Here's how the part is built. I have some questions about the finished solid (model axes, mm). Face numbers are marked on the shaded views. A direction names the side the tool comes from. Coordinates: 2 decimals unless noted, no trailing zeros. Loops run counter-clockwise (first coordinate to the right, second up) from the corner with the lowest first, then second, coordinate; pieces in that order, holes last. Notation, with made-up numbers: M -35.5,-21.75 L -17.5,-21.75 A28 ccw -17.5,-2.75 Z; hole C 64.25,54.5 d5. An arc over 180 degrees is marked long. Use CSV: the item, a comma, the result in double quotes. Start each with the question number.
Q1. If we section it at D-D (z = 9.5): State how many separate pieces and enclosed holes the cut face has, and give its area (3 significant figures).
Q2. Which directions (+Z, -Z, +X, -X, +Y, -Y) give clear straight access to the entire face, cutting with the end or side of a thin tool? Please do the marked faces 1 and 2.
Q3. For pin 1 Ø12 at (x, y) = (-23, -35.5) entering from -Z; pin 2 Ø0.6 at (x, z) = (-45.5, 20) entering from -Y (3 decimals); pin 3 Ø0.8 at (y, z) = (-37.5, 11) entering from -X (3 decimals), each with a flat end and sliding along its axis, tell me the tip position at first contact or that it passes through.
Q4. If we section it at B-B (y = -53.65): Please give me the cut outline in (x, z) (3 decimals).
Q5. If we section it at C-C (x = -17): Please give me the cut outline in (y, z), and give its area (3 significant figures).
Q6. If we section it at A-A (x = 32): Please give me the cut outline in (y, z), and give its area (3 significant figures).
Q7. Please list where these lines run through material, in increasing order: probe 1 along X at (y, z) = (-30, 16.5) (3 decimals); probe 2 along X at (y, z) = (-53, 20) (3 decimals); probe 3 along Y at (x, z) = (19, 4). Write a range as [from, to].
Q8. If we mould it in two halves opening along X, with no side actions, what happens to the marked faces 3, 4 and 5? For each: +X half, -X half, draft (parallel to the pull), parting line (faces both ways), or undercut.
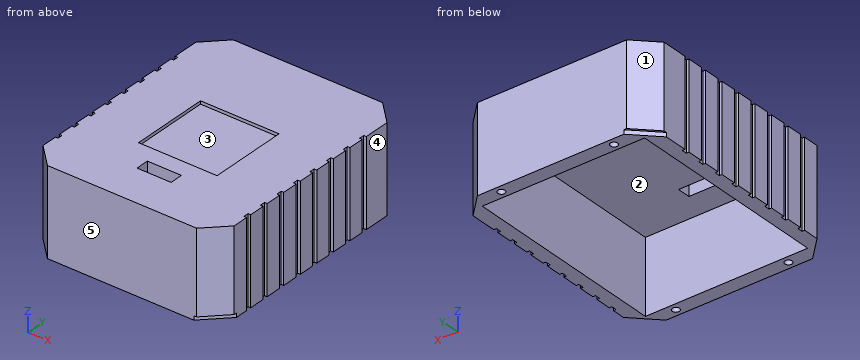
from build123d import *

# Parameters (mm, degrees)
SKETCH1_W           = 92.71
SKETCH1_H           = 114.3
BOSS_EXTRUDE1_DEPTH = 41.91
SKETCH2_W           = 2.54
SKETCH2_H           = 2.54
CUT_EXTRUDE1_DEPTH  = 85.683862837
CHAMFER1_SIZE       = 10.16
SKETCH3_R           = 1.750000056
CUT_EXTRUDE2_DEPTH  = 25.4
SKETCH4_W           = 78.71
SKETCH4_H           = 100.30000006
CUT_EXTRUDE3_DEPTH  = 35.56
SKETCH6_W           = 16.51
SKETCH6_H           = 6.35
CUT_EXTRUDE5_DEPTH  = 85.683862837
CUT_EXTRUDE6_DEPTH  = 2
SKETCH8_W           = 38.1
SKETCH8_H           = 38.1
CUT_EXTRUDE7_DEPTH  = 1.5


with BuildPart() as part:
    # Sketch1 → Boss-Extrude1 (new body)
    with BuildSketch(Plane.XY):
        Rectangle(SKETCH1_W, SKETCH1_H)
    extrude(amount=BOSS_EXTRUDE1_DEPTH)

    # Sketch2 → Cut-Extrude1 (cut, through all)
    with BuildSketch(Plane(origin=(0, 0, 0), x_dir=(-1, 0, 0), z_dir=(0, 0, -1))):
        with Locations((-46.355, -38.1)):
            Rectangle(SKETCH2_W, SKETCH2_H)
        with Locations((46.355, -38.1)):
            Rectangle(SKETCH2_W, SKETCH2_H)
        with Locations((-46.355, -27.94)):
            Rectangle(SKETCH2_W, SKETCH2_H)
        with Locations((46.355, -27.94)):
            Rectangle(SKETCH2_W, SKETCH2_H)
        with Locations((-46.355, -17.78)):
            Rectangle(SKETCH2_W, SKETCH2_H)
        with Locations((46.355, -17.78)):
            Rectangle(SKETCH2_W, SKETCH2_H)
        with Locations((-46.355, -7.62)):
            Rectangle(SKETCH2_W, SKETCH2_H)
        with Locations((46.355, -7.62)):
            Rectangle(SKETCH2_W, SKETCH2_H)
        with Locations((-46.355, 2.54)):
            Rectangle(SKETCH2_W, SKETCH2_H)
        with Locations((46.355, 2.54)):
            Rectangle(SKETCH2_W, SKETCH2_H)
        with Locations((-46.355, 12.7)):
            Rectangle(SKETCH2_W, SKETCH2_H)
        with Locations((46.355, 12.7)):
            Rectangle(SKETCH2_W, SKETCH2_H)
        with Locations((-46.355, 22.86)):
            Rectangle(SKETCH2_W, SKETCH2_H)
        with Locations((46.355, 22.86)):
            Rectangle(SKETCH2_W, SKETCH2_H)
        with Locations((-46.355, 33.02)):
            Rectangle(SKETCH2_W, SKETCH2_H)
        with Locations((46.355, 33.02)):
            Rectangle(SKETCH2_W, SKETCH2_H)
    extrude(amount=-CUT_EXTRUDE1_DEPTH, mode=Mode.SUBTRACT)

    # Chamfer1
    chamfer1_edges = [part.edges().sort_by_distance(p)[0] for p in [
        (46.355, -57.15, 20.955),
        (-46.355, -57.15, 20.955),
        (-46.355, 57.15, 20.955),
        (46.355, 57.15, 20.955),
    ]]
    chamfer(chamfer1_edges, length=CHAMFER1_SIZE)

    # Sketch3 → Cut-Extrude2 (cut)
    with BuildSketch(Plane(origin=(0, 0, 0), x_dir=(-1, 0, 0), z_dir=(0, 0, -1))):
        with Locations((-27.305, -53.649999888)):
            Circle(SKETCH3_R)
        with Locations((-27.305, 53.65)):
            Circle(SKETCH3_R)
        with Locations((27.305, 53.649999888)):
            Circle(SKETCH3_R)
        with Locations((27.305, -53.649999888)):
            Circle(SKETCH3_R)
    extrude(amount=-CUT_EXTRUDE2_DEPTH, mode=Mode.SUBTRACT)

    # Sketch4 → Cut-Extrude3 (cut)
    with BuildSketch(Plane(origin=(0, 0, 0), x_dir=(-1, 0, 0), z_dir=(0, 0, -1))):
        Rectangle(SKETCH4_W, SKETCH4_H)
    extrude(amount=-CUT_EXTRUDE3_DEPTH, mode=Mode.SUBTRACT)

    # Sketch6 → Cut-Extrude5 (cut, through all)
    with BuildSketch(Plane.XY.offset(41.91)):
        with Locations((0, -34.29)):
            Rectangle(SKETCH6_W, SKETCH6_H)
    extrude(amount=-CUT_EXTRUDE5_DEPTH, mode=Mode.SUBTRACT)

    # Sketch7 → Cut-Extrude6 (cut)
    with BuildSketch(Plane(origin=(0, 0, 0), x_dir=(-1, 0, 0), z_dir=(0, 0, -1))):
        Polygon((40.567893219, 51.362893219), (46.355, 45.575786438), (46.355, 46.99), (36.195, 57.15), (34.780786438, 57.15), align=None)
        Polygon((-40.567893219, -51.362893219), (-46.355, -45.575786438), (-46.355, -46.99), (-36.195, -57.15), (-34.780786438, -57.15), align=None)
    extrude(amount=-CUT_EXTRUDE6_DEPTH, mode=Mode.SUBTRACT)

    # Sketch8 → Cut-Extrude7 (cut)
    with BuildSketch(Plane.XY.offset(41.91)):
        with Locations((0, -3.81)):
            Rectangle(SKETCH8_W, SKETCH8_H)
    extrude(amount=-CUT_EXTRUDE7_DEPTH, mode=Mode.SUBTRACT)


solid = part.part
Results below:
1,separate pieces,"1"
1,enclosed holes,"5"
1,area,"2,410 mm^2"
2,face 1,"+Z, -Z, -X, +Y"
2,face 2,"-Z"
3,pin 1,"z = 35.56"
3,pin 2,"y = -48.145"
3,pin 3,"x = -45.085"
4,outline,"M -39.695,0 L -29.055,0 L -29.055,25.4 L -25.555,25.4 L -25.555,0 L 25.555,0 L 25.555,25.4 L 29.055,25.4 L 29.055,0 L 38.281,0 L 38.281,2 L 39.695,2 L 39.695,41.91 L -39.695,41.91 Z"
5,outline,"M -57.15,0 L -50.15,0 L -50.15,35.56 L 50.15,35.56 L 50.15,0 L 57.15,0 L 57.15,41.91 L 15.24,41.91 L 15.24,40.41 L -22.86,40.41 L -22.86,41.91 L -57.15,41.91 Z"
5,area,"1,170 mm^2"
6,outline,"M -57.15,0 L -50.15,0 L -50.15,35.56 L 50.15,35.56 L 50.15,0 L 57.15,0 L 57.15,41.91 L -57.15,41.91 Z"
6,area,"1,220 mm^2"
7,probe 1,"[-46.355, -39.355], [39.355, 46.355]"
7,probe 2,"[-40.345, -28.93], [-25.68, 25.68], [28.93, 40.345]"
7,probe 3,"[-57.15, -50.15], [50.15, 57.15]"
8,face 3,"undercut"
8,face 4,"+X half"
8,face 5,"draft"
